from build123d import *

# Parameters (mm, degrees)
SKETCH1_W           = 62.484
SKETCH1_H           = 43.18
SKETCH1_R           = 2.4003
BOSS_EXTRUDE1_DEPTH = 7.62
SKETCH2_W           = 41.91
SKETCH2_H           = 43.007401248
BOSS_EXTRUDE2_DEPTH = 0.762


with BuildPart() as part:
    # Sketch1 → Boss-Extrude1 (new body)
    with BuildSketch(Plane(origin=(0, 0, 0), x_dir=(1, 0, 0), z_dir=(0, 1, 0))):
        with Locations((0, 0.086299376)):
            Rectangle(SKETCH1_W, SKETCH1_H)
        with Locations(Location((-26.162, 15.326299376, 0), (0, 0, 90))):
            Circle(SKETCH1_R, mode=Mode.SUBTRACT)
        with Locations(Location((-26.162, -15.153700624, 0), (0, 0, 90))):
            Circle(SKETCH1_R, mode=Mode.SUBTRACT)
        with Locations(Location((26.162, -15.153700624, 0), (0, 0, 90))):
            Circle(SKETCH1_R, mode=Mode.SUBTRACT)
        with Locations(Location((26.162, 15.326299376, 0), (0, 0, 90))):
            Circle(SKETCH1_R, mode=Mode.SUBTRACT)
    extrude(amount=BOSS_EXTRUDE1_DEPTH)

    # Sketch2 → Boss-Extrude2 (add)
    with BuildSketch(Plane.XZ):
        Rectangle(SKETCH2_W, SKETCH2_H)
    extrude(amount=BOSS_EXTRUDE2_DEPTH)


solid = part.part
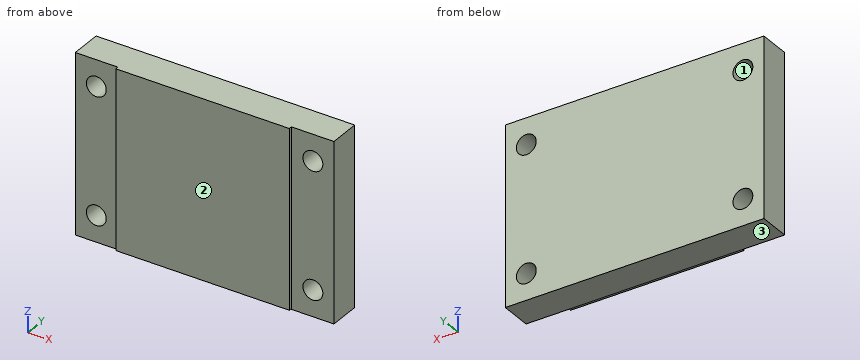
Geometry check sheet. Reference: the model listing, model coordinates, mm. Face numbers are marked on the shaded views. Give positions to 0.01 mm unless a question says otherwise; leave off trailing zeros. Loops run counter-clockwise (first coordinate to the right, second up) from the corner with the lowest first, then second, coordinate; pieces in that order, holes last. Notation, with made-up numbers: (-34, 24) -> (19, 24) arc R18 ccw to (19, 40) -> close; hole circle Ø9 at (28.5, 52). An arc over 180 degrees is marked (long way). Answer in a Markdown table with one row per item. Add a question column.
1) Cross-section at A-A on z = -15.5. Record the boundary of the cut face in (x, y) (3 decimals), and give its area (3 significant figures).
2) Cross-section at C-C on z = 8.5. Record the boundary of the cut face in (x, y) (3 decimals).
3) Material ranges on probe 1 along Z at (x, y) = (-26, 4.5); probe 2 along X at (y, z) = (2, 14); probe 3 along X at (y, z) = (5.5, -14), recorded low to high. Write a range as from..to.
4) Draft check along Z on the marked faces 1, 2 and 3. Enter one of: pulls with the +Z half, pulls with the -Z half, needs draft (parallel to the pull), parting line crosses it, or undercut.
5) Gauge pin test, flat ends, axial feed: P1, Ø0.8, axis at x = 3.5, y = -0.5, coming from the -Z side; P2, Ø0.6, axis at y = -0.5, z = 9, coming from the -X side (3 decimals); P3, Ø0.6, axis at y = -0.5, z = 10, coming from the +X side (3 decimals). Record the tip position at first contact, or that the pin passes through.
6) Cross-section at D-D on x = -23. Record the boundary of the cut face in (y, z).
7) Cross-section at B-B on y = 1. Record the boundary of the cut face in (x, z), and give its area (3 significant figures).
Outcome:
| question | item | result |
|---|---|---|
| 1 | outline | (-31.242, 0) -> (-28.556, 0) -> (-28.556, 7.62) -> (-31.242, 7.62) -> close; (-23.768, 0) -> (-20.955, 0) -> (-20.955, -0.762) -> (20.955, -0.762) -> (20.955, 0) -> (23.768, 0) -> (23.768, 7.62) -> (-23.768, 7.62) -> close; (28.556, 0) -> (31.242, 0) -> (31.242, 7.62) -> (28.556, 7.62) -> close |
| 1 | area | 435 mm^2 |
| 2 | outline | (-31.242, 0) -> (-20.955, 0) -> (-20.955, -0.762) -> (20.955, -0.762) -> (20.955, 0) -> (31.242, 0) -> (31.242, 7.62) -> (-31.242, 7.62) -> close |
| 3 | probe 1 | z = -21.68..-17.72, -12.93..12.76, 17.55..21.5 |
| 3 | probe 2 | x = -31.24..-28.27, -24.06..24.06, 28.27..31.24 |
| 3 | probe 3 | x = -31.24..-28.16, -24.16..24.16, 28.16..31.24 |
| 4 | face 1 | undercut |
| 4 | face 2 | needs draft |
| 4 | face 3 | pulls with the -Z half |
| 5 | P1 | stops at z = -21.5 |
| 5 | P2 | stops at x = -20.955 |
| 5 | P3 | stops at x = 20.955 |
| 6 | outline | (0, -21.68) -> (7.62, -21.68) -> (7.62, 21.5) -> (0, 21.5) -> close |
| 7 | outline | (-31.24, -21.68) -> (31.24, -21.68) -> (31.24, 21.5) -> (-31.24, 21.5) -> close; hole circle Ø4.8 at (-26.16, -15.33); hole circle Ø4.8 at (-26.16, 15.15); hole circle Ø4.8 at (26.16, -15.33); hole circle Ø4.8 at (26.16, 15.15) |
| 7 | area | 2,630 mm^2 |
